Print and shaded views of the part. All mm, measured from the part's lowest x, y and z. A direction names the side the tool comes from. Give positions to 0.01 mm unless a question says otherwise; leave off trailing zeros. Loops run counter-clockwise (first coordinate to the right, second up) from the corner with the lowest first, then second, coordinate; pieces in that order, holes last. Notation, with made-up numbers: (-38, 2.25) - (4, 2.25) arc R28 cw to (4, 31.25) - close; hole circle Ø4 at (24, 7.5). An arc over 180 degrees is marked (long way). Return JSON: item names as keys, results as strings.
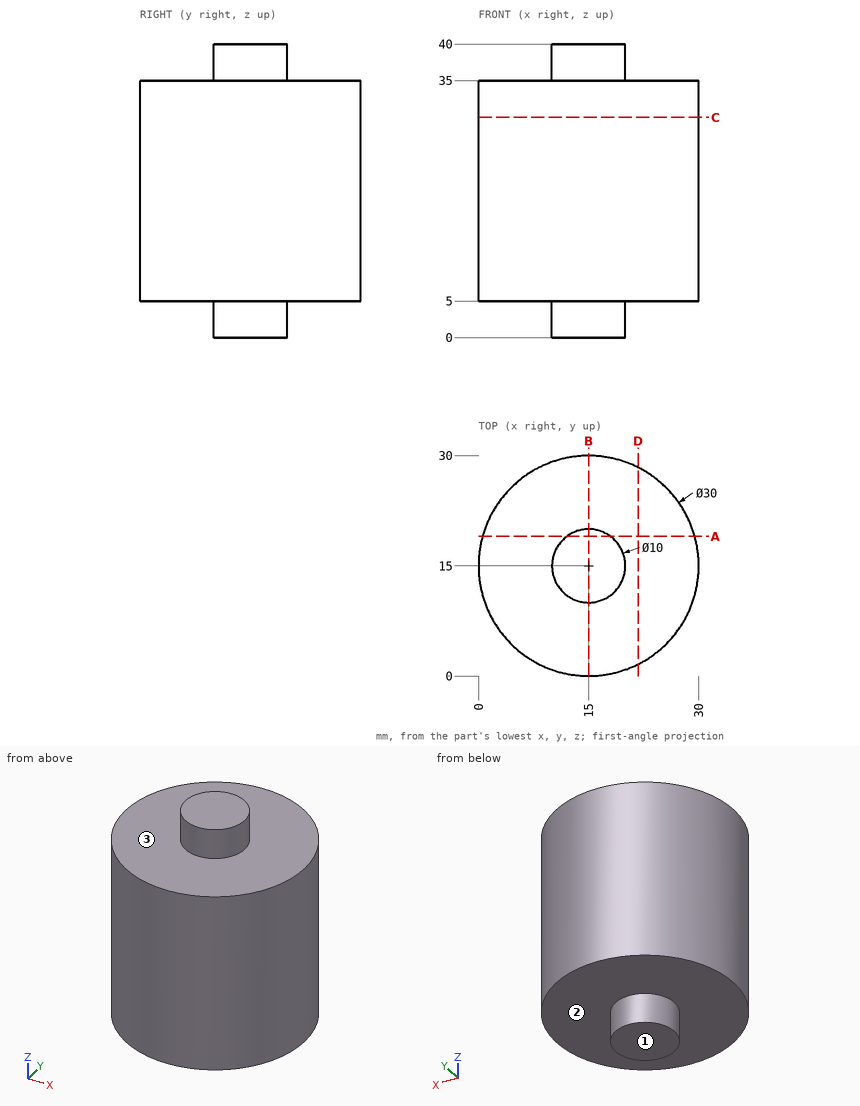
1. Which spindle directions (+Z, -Z, +X, -X, +Y, -Y) get a long thin tool onto all of the face, cutting with end or side? Do the marked faces 1, 2 and 3. Say none if no direction does.
Values follow:
{"face 1": "-Z, +X, -X, +Y, -Y", "face 2": "-Z", "face 3": "+Z"}
2. Cut at C-C, the plane z = 30. Write the cut outline in (x, y), plus the area to 3 significant figures.
Values follow:
{"outline": "circle Ø30 at (15, 15)", "area": "707 mm²"}
3. Cut at B-B, the plane x = 15. Write the cut outline in (y, z), plus the area to 3 significant figures.
Values follow:
{"outline": "(0, 5) - (10, 5) - (10, 0) - (20, 0) - (20, 5) - (30, 5) - (30, 35) - (20, 35) - (20, 40) - (10, 40) - (10, 35) - (0, 35) - close", "area": "1,000 mm²"}
4. Drop flat-ended pins along their axis: P1, Ø3, axis at x = 7, z = 4.5, coming from the +Y side; P2, Ø6, axis at x = 3.5, y = 23, coming from the +Z side; P3, Ø6, axis at y = 11.5, z = 5.5, coming from the +X side. Give the stop position or say it passes through.
Values follow:
{"P1": "stops at y = 28.48", "P2": "stops at z = 35", "P3": "stops at x = 29.99"}
5. Cut at A-A, the plane y = 19. Write the cut outline in (x, z), plus the area to 3 significant figures.
Values follow:
{"outline": "(0.54, 5) - (12, 5) - (12, 0) - (18, 0) - (18, 5) - (29.46, 5) - (29.46, 35) - (18, 35) - (18, 40) - (12, 40) - (12, 35) - (0.54, 35) - close", "area": "927 mm²"}
6. Cut at D-D, the plane x = 21.75. Write the cut outline in (y, z).
Values follow:
{"outline": "(1.6, 5) - (28.4, 5) - (28.4, 35) - (1.6, 35) - close"}
7. Drill centre lines: probe 1 along Z at (x, y) = (2.75, 8); probe 2 along X at (y, z) = (14.75, 29.5); probe 3 along X at (y, z) = (2, 20). Where is each one in solid material? Low to high.
Values follow:
{"probe 1": "z = 5 to 35", "probe 2": "x = 0 to 30", "probe 3": "x = 7.52 to 22.48"}
